Work out the finished part from the listing and answer in its coordinate system (mm). Coordinates: 2 decimals unless noted, no trailing zeros. Order: outer loops, then holes, each group sorted by start corner. A loop starts at its lowest first (then second) coordinate and runs counter-clockwise, first axis right, second up. Notation, with made-up numbers: M -26.75,14.25 L 32.25,14.25 A24 cw 32.25,48.25 Z; hole C 64,30 d3. An arc over 180 degrees is marked long. Use a Markdown table: item, result.
from build123d import *

# Parameters (mm, degrees)
SKETCH1_R           = 10
SKETCH1_R_2         = 3
BOSS_EXTRUDE1_DEPTH = 5


with BuildPart() as part:
    # Sketch1 → Boss-Extrude1 (new, symmetric)
    with BuildSketch(Plane.XY):
        with BuildLine():
            ThreePointArc((37.492992706, -7.419029226), (42.5, 0), (37.492992706, 7.419029226))
            ThreePointArc((37.492992706, 7.419029226), (27.654966395, 15.966602293), (25.171564134, 28.760369534))
            ThreePointArc((25.171564134, 28.760369534), (21.25, 36.806079661), (12.321428571, 36.17939876))
            ThreePointArc((12.321428571, 36.17939876), (0, 31.933204585), (-12.321428571, 36.17939876))
            ThreePointArc((-12.321428571, 36.17939876), (-21.25, 36.806079661), (-25.171564134, 28.760369534))
            ThreePointArc((-25.171564134, 28.760369534), (-27.654966395, 15.966602293), (-37.492992706, 7.419029226))
            ThreePointArc((-37.492992706, 7.419029226), (-42.5, 0), (-37.492992706, -7.419029226))
            ThreePointArc((-37.492992706, -7.419029226), (-27.654966395, -15.966602293), (-25.171564134, -28.760369534))
            ThreePointArc((-25.171564134, -28.760369534), (-21.25, -36.806079661), (-12.321428571, -36.17939876))
            ThreePointArc((-12.321428571, -36.17939876), (0, -31.933204585), (12.321428571, -36.17939876))
            ThreePointArc((12.321428571, -36.17939876), (21.25, -36.806079661), (25.171564134, -28.760369534))
            ThreePointArc((25.171564134, -28.760369534), (27.654966395, -15.966602293), (37.492992706, -7.419029226))
        make_face()
        Circle(SKETCH1_R, mode=Mode.SUBTRACT)
        with Locations((34.5, 0)):
            Circle(SKETCH1_R_2, mode=Mode.SUBTRACT)
        with Locations((17.25, -29.877876431)):
            Circle(SKETCH1_R_2, mode=Mode.SUBTRACT)
        with Locations((-17.25, -29.877876431)):
            Circle(SKETCH1_R_2, mode=Mode.SUBTRACT)
        with Locations((-34.5, 0)):
            Circle(SKETCH1_R_2, mode=Mode.SUBTRACT)
        with Locations((-17.25, 29.877876431)):
            Circle(SKETCH1_R_2, mode=Mode.SUBTRACT)
        with Locations((17.25, 29.877876431)):
            Circle(SKETCH1_R_2, mode=Mode.SUBTRACT)
    extrude(amount=BOSS_EXTRUDE1_DEPTH, both=True)


solid = part.part
1. Section D-D on z = 3.5 is taken. Determine the outline of the cut face in (x, y).
Answers below:
| item | result |
|---|---|
| outline | M -37.49,-7.42 A20 cw -25.17,-28.76 A8 ccw -12.32,-36.18 A20 cw 12.32,-36.18 A8 ccw 25.17,-28.76 A20 cw 37.49,-7.42 A8 ccw 37.49,7.42 A20 cw 25.17,28.76 A8 ccw 12.32,36.18 A20 cw -12.32,36.18 A8 ccw -25.17,28.76 A20 cw -37.49,7.42 A8 ccw Z; hole C -34.5,0 d6; hole C -17.25,-29.88 d6; hole C -17.25,29.88 d6; hole C 0,0 d20; hole C 17.25,-29.88 d6; hole C 17.25,29.88 d6; hole C 34.5,0 d6 |
2. Section A-A on y = 0 is taken. Determine the outline of the cut face in (x, z), then the cut area to 3 significant figures.
Answers below:
| item | result |
|---|---|
| outline | M -42.5,-5 L -37.5,-5 L -37.5,5 L -42.5,5 Z; M -31.5,-5 L -10,-5 L -10,5 L -31.5,5 Z; M 10,-5 L 31.5,-5 L 31.5,5 L 10,5 Z; M 37.5,-5 L 42.5,-5 L 42.5,5 L 37.5,5 Z |
| area | 530 mm² |
3. Flat-ended cylindrical pins translate along their axes: P1, Ø2, axis at y = 25, z = 1.5, coming from the +X side; P2, Ø4, axis at x = -22, z = 0, coming from the +Y side; P3, Ø3, axis at x = -20.5, z = 3.5, coming from the -Y side. Find the tip coordinate at first contact, or state that the pin passes through.
Answers below:
| item | result |
|---|---|
| P1 | x = 25.07 |
| P2 | y = 37.39 |
| P3 | y = -37.68 |
4. Find the intervals of material crossed by probe 1 along Y at (x, z) = (17.25, 0.75); probe 2 along X at (y, z) = (-30.5, 3); probe 3 along Y at (x, z) = (19, -1), in increasing order.
Answers below:
| item | result |
|---|---|
| probe 1 | -37.88 to -32.88, -26.88 to 26.88, 32.88 to 37.88 |
| probe 2 | -25.23 to -20.18, -14.32 to 14.32, 20.18 to 25.23 |
| probe 3 | -37.68 to -32.31, -27.44 to 27.44, 32.31 to 37.68 |
5. For a pull along X with two mould halves and no side action, classify faces 1 (the face through (-27.56, 16.13, 0.07)), 2 (the face through (-10, -8, 5)), 3 (the face through (-0.186, -31.934, 0.07)), 4 (the face through (27.749, 15.806, 0.07)) as +X half, -X half, draft (parallel to the pull), parting line (faces both ways), or undercut.
Answers below:
| item | result |
|---|---|
| face 1 | -X half |
| face 2 | draft |
| face 3 | undercut |
| face 4 | +X half |
6. Section C-C on x = -7.5 is taken. Determine the outline of the cut face in (y, z), then the cut area to 3 significant figures.
Answers below:
| item | result |
|---|---|
| outline | M -33.39,-5 L -6.61,-5 L -6.61,5 L -33.39,5 Z; M 6.61,-5 L 33.39,-5 L 33.39,5 L 6.61,5 Z |
| area | 536 mm² |
7. Section B-B on x = 17.25 is taken. Determine the outline of the cut face in (y, z), then the cut area to 3 significant figures.
Answers below:
| item | result |
|---|---|
| outline | M -37.88,-5 L -32.88,-5 L -32.88,5 L -37.88,5 Z; M -26.88,-5 L 26.88,-5 L 26.88,5 L -26.88,5 Z; M 32.88,-5 L 37.88,-5 L 37.88,5 L 32.88,5 Z |
| area | 638 mm² |
